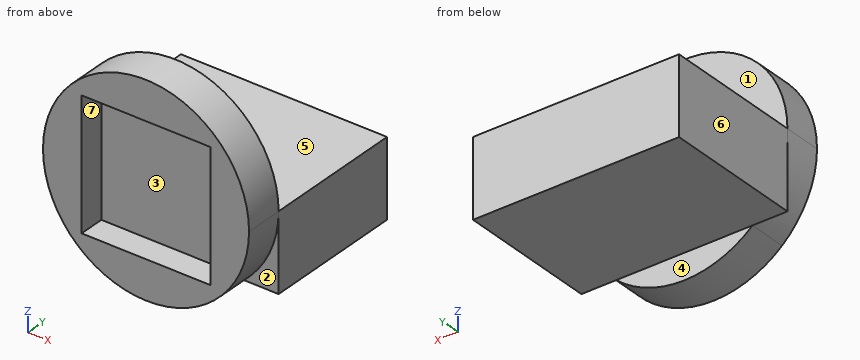
from build123d import *

# Parameters (mm, degrees)
F1_DEPTH = 11
F2_DEPTH = 3
F3_W     = 10
F3_H     = 10
F4_DEPTH = 2


with BuildPart() as f1:
    # F0 (on Front) → F1 (new body)
    with BuildSketch(Plane.XZ):
        with BuildLine():
            ThreePointArc((-5.2915026221, -6), (-7.2915026221, -3.2915026221), (-8, 0))
            Line((-8, 0), (-8, -6))
            Line((-8, -6), (-5.2915026221, -6))
        make_face()
        with BuildLine():
            Line((8, -6), (8, 0))
            ThreePointArc((8, 0), (7.2915026221, -3.2915026221), (5.2915026221, -6))
            Line((5.2915026221, -6), (8, -6))
        make_face()
        with BuildLine():
            ThreePointArc((5.2915026221, -6), (7.2915026221, -3.2915026221), (8, 0))
            Line((8, 0), (-8, 0))
            ThreePointArc((-8, 0), (-7.2915026221, -3.2915026221), (-5.2915026221, -6))
            Line((-5.2915026221, -6), (5.2915026221, -6))
        make_face()
    extrude(amount=-F1_DEPTH)

    # F0 (on Front) → F2 (join)
    with BuildSketch(Plane.XZ):
        with BuildLine():
            Line((-8, 0), (8, 0))
            ThreePointArc((8, 0), (0, 8), (-8, 0))
        make_face()
        with BuildLine():
            ThreePointArc((5.2915026221, -6), (7.2915026221, -3.2915026221), (8, 0))
            Line((8, 0), (-8, 0))
            ThreePointArc((-8, 0), (-7.2915026221, -3.2915026221), (-5.2915026221, -6))
            Line((-5.2915026221, -6), (5.2915026221, -6))
        make_face()
        with BuildLine():
            ThreePointArc((-5.2915026221, -6), (0, -8), (5.2915026221, -6))
            Line((5.2915026221, -6), (-5.2915026221, -6))
        make_face()
    extrude(amount=F2_DEPTH)

    # F3 (on face) → F4 (cut)
    with BuildSketch(Plane.XZ.offset(3)):
        Rectangle(F3_W, F3_H)
    extrude(amount=-F4_DEPTH, mode=Mode.SUBTRACT)


solid = f1.part
For this review, take the finished solid that the model builds, in its own axes (mm). Face numbers are marked on the shaded views. A direction names the side the tool comes from. Give positions to 0.01 mm unless a question says otherwise; leave off trailing zeros. Loops run counter-clockwise (first coordinate to the right, second up) from the corner with the lowest first, then second, coordinate; pieces in that order, holes last. Notation, with made-up numbers: M -2.75,-16 L 46.25,-16 A17 ccw 46.25,5 Z; hole C 66.25,87 d7. An arc over 180 degrees is marked long. Put each result on its own line as item: value. Start each with the question number.
(1) Wall thickness on L1, parallel to Z at x = -2, y = 9.25; L2, parallel to Y at x = -1.5, z = -1.75; L3, parallel to Y at x = 2.75, z = 1.5: over which ranges is each line inside the solid? List them lowest first.
(2) Add section D-D, the plane y = 8. Write out the cut boundary in (x, z).
(3) Add section C-C, the plane z = -4.5. Write out the cut boundary in (x, y), then the cut area to 3 significant figures.
(4) The part is to be moulded in two halves that separate along X. For the marked faces 5, 6 and 7, say which applies: +X half, -X half, draft (parallel to the pull), parting line (faces both ways), or undercut.
(5) Add section B-B, the plane x = 0. Write out the cut boundary in (y, z), then the cut area to 3 significant figures.
(6) Machinability: for the marked faces 1, 2, 3 and 4, which of the approach directions +Z, -Z, +X, -X, +Y, -Y give a long, thin tool a straight path to every point of the face, cutting with its end or side? Answer none if there is none.
(7) Add section A-A, the plane y = -1.5. Write out the cut boundary in (x, z), then the cut area to 3 significant figures.
(8) For pin 1 (2 mm diameter, centred on x = -1, z = -0.5, fed in from -Y); pin 2 (1 mm diameter, centred on x = 0.5, y = 3, fed in from -Z); pin 3 (5 mm diameter, centred on y = -1, z = 3.5, fed in from -X), all flat-tipped, find the tip position at first contact; note any pin that passes through.
Result:
1. L1: z = -6 to 0
1. L2: y = -1 to 11
1. L3: y = -1 to 0
2. outline: M -8,-6 L 8,-6 L 8,0 L -8,0 Z
3. outline: M -8,0 L -6.61,0 L -6.61,-3 L -5,-3 L -5,-1 L 5,-1 L 5,-3 L 6.61,-3 L 6.61,0 L 8,0 L 8,11 L -8,11 Z
3. area: 196 mm^2
4. face 5: draft
4. face 6: -X half
4. face 7: undercut
5. outline: M -3,-8 L 0,-8 L 0,-6 L 11,-6 L 11,0 L 0,0 L 0,8 L -3,8 L -3,5 L -1,5 L -1,-5 L -3,-5 Z
5. area: 94.0 mm^2
6. face 1: +Z, +X, -X, +Y
6. face 2: -Z, +X, -Y
6. face 3: -Y
6. face 4: -Z, +X, -X, +Y
7. outline: C 0,0 d16; hole M -5,-5 L 5,-5 L 5,5 L -5,5 Z
7. area: 101 mm^2
8. pin 1: stops at y = -1
8. pin 2: stops at z = -6
8. pin 3: stops at x = -7.94
